from build123d import *

# Parameters (mm, degrees)
F2_R     = 20.330932
F3_DEPTH = 76.2


with BuildPart() as f1:
    # F0 (on Top) → F1 (revolve)
    with BuildSketch(Plane.XY):
        Polygon((34.927377, 46.017325), (0, 2.195979), (-21.864308, 2.195979), (-21.864308, -9.834165), (0, -9.834165), (0, 0), (35.994954, 45.160774), align=None)
    revolve(axis=Axis((-21.864308, -3.819093, 0), (0, -1, 0)))

    # F2 (on face) → F3 (cut)
    with BuildSketch(Plane.XZ.offset(9.834165)):
        with Locations((-21.864308, 0)):
            Circle(F2_R)
    extrude(amount=-F3_DEPTH, mode=Mode.SUBTRACT)


solid = f1.part
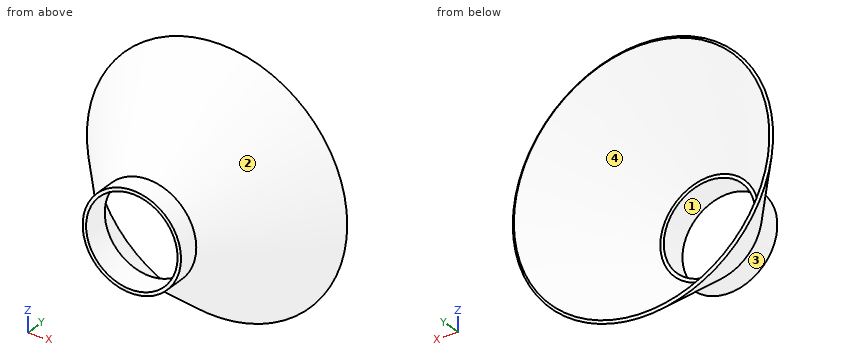
The model under review builds one solid part; all positions refer to its coordinate system, in mm. Face numbers are marked on the shaded views. A direction names the side the tool comes from. Round coordinates to 2 decimals unless told otherwise and drop trailing zeros. Write each loop counter-clockwise with the first axis right and the second up, starting at its lowest first coordinate (ties: lowest second). Pieces come first, ordered by that corner, then holes. Notation, with made-up numbers: (3.25, 78.5) - (10.25, 78.5) arc R22 ccw to (10.25, 114.5) - close; hole circle Ø4 at (-21, -27). An arc over 180 degrees is marked (long way). One line per item, written item: value. Start each with the question number.
1. Clearance check with flat-ended pins moving along their axes: P1, Ø3, axis at y = 37.5, z = 20.5, coming from the +X side; P2, Ø2, axis at y = 23.5, z = 3.5, coming from the -X side; P3, Ø1, axis at x = -8.5, y = 33, coming from the -Z side. State where each tip first meets the part, or that it passes through.
2. Consider section C-C on y = 42. Write out the cut boundary in (x, z), and give its area (3 significant figures).
3. To check wall thickness, follow L1, parallel to Z at x = -19.5, y = 27; L2, parallel to Z at x = 19, y = 40; L3, parallel to X at y = 30.5, z = -19. State the ranges of each line that lie inside material, in increasing order. Write a range as from..to.
4. Machinability: for the marked faces 3 and 4, which of the approach directions +Z, -Z, +X, -X, +Y, -Y give a long, thin tool a straight path to every point of the face, cutting with its end or side? Answer none if there is none.
5. The part is to be moulded in two halves that separate along Z. For the marked faces 1 and 2, say which applies: released by +Z, released by -Z, zero draft, split by the parting line, or undercut.
6. Consider section A-A on z = 0. Write out the cut boundary in (x, y), and give its area (3 significant figures).
7. Consider section B-B on y = 22. Write out the cut boundary in (x, z), and give its area (3 significant figures).
Checks:
1. P1: stops at x = 27.1
1. P2: stops at x = -63.11
1. P3: stops at z = -46.71
2. outline: circle Ø110.68 at (-21.86, 0); hole circle Ø107.18 at (-21.86, 0)
2. area: 599 mm^2
3. L1: z = -43.32..-41.57, 41.57..43.32
3. L2: z = -34.91..-32.15, 32.15..34.91
3. L3: x = -63.95..-62.02, 18.29..20.22
4. face 3: -Y
4. face 4: +Y
5. face 1: undercut
5. face 2: split by the parting line
6. outline: (-79.72, 45.16) - (-43.73, 0) - (-43.73, -9.83) - (-42.2, -9.83) - (-42.2, 2.2) - (-43.73, 2.2) - (-78.66, 46.02) - close; (-1.53, -9.83) - (0, -9.83) - (0, 0) - (35.99, 45.16) - (34.93, 46.02) - (0, 2.2) - (-1.53, 2.2) - close
6. area: 193 mm^2
7. outline: circle Ø78.8 at (-21.86, 0); hole circle Ø75.3 at (-21.86, 0)
7. area: 424 mm^2
